Part print with two shaded views. Sizes in mm from the minimum x, y, z corner. Round coordinates to 2 decimals unless told otherwise and drop trailing zeros. Write each loop counter-clockwise with the first axis right and the second up, starting at its lowest first coordinate (ties: lowest second). Pieces come first, ordered by that corner, then holes. Notation, with made-up numbers: (-14, -29) - (-1, -29) arc R18 ccw to (-1, -19) - close; hole circle Ø4 at (56, 55.25). An arc over 180 degrees is marked (long way). Use one line per item in the form item = value. Start each with the question number.
Item 1: Drill centre lines: L1, parallel to Z at x = 125, y = 4.25; L2, parallel to X at y = 12, z = 80.5; L3, parallel to Z at x = 73, y = 8.5. Where is each one in solid material? Low to high.
Item 2: Band-saw the part on A-A, the plane z = 80.5. List the corners of the cut face in (x, y), and give its area (3 significant figures).
Item 3: Pin check, flat tips, straight feed: pin 1 (5 mm diameter, centred on y = 3, z = 27.5, fed in from -X); pin 2 (9.5 mm diameter, centred on x = 125, z = 80.5, fed in from -Y); pin 3 (3.5 mm diameter, centred on x = 125, z = 19.5, fed in from +Y). Stop position of each tip, or through.
Item 4: Band-saw the part on B-B, the plane x = 75. List the corners of the cut face in (y, z), and give its area (3 significant figures).
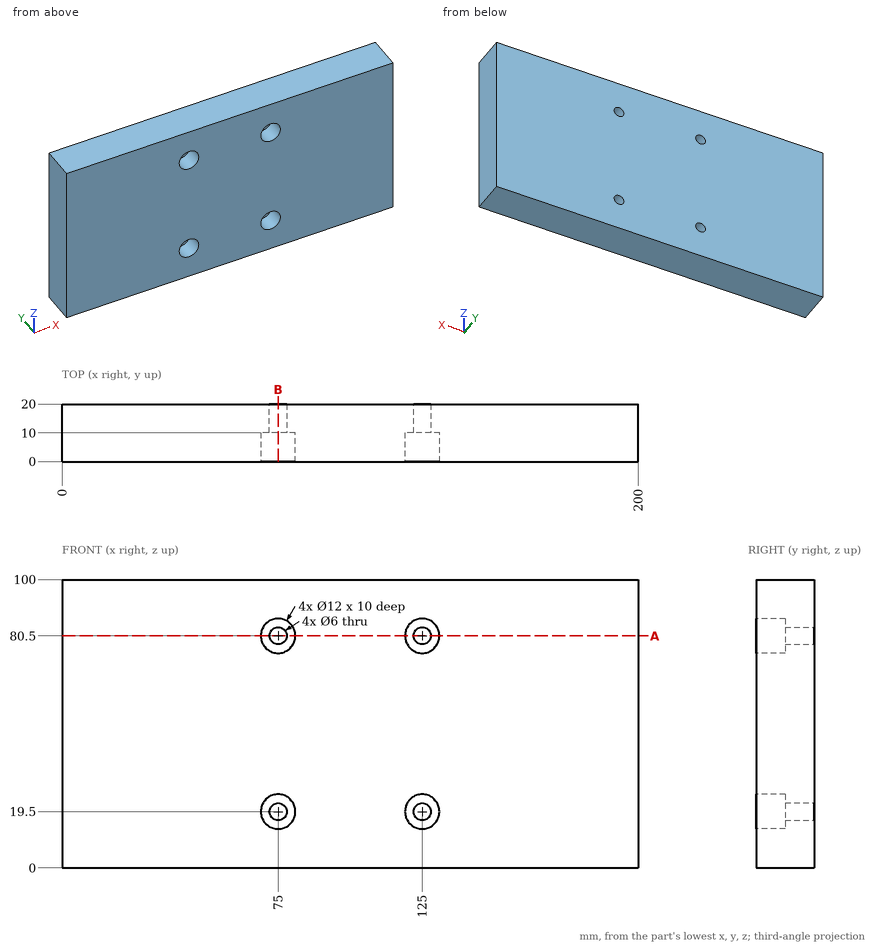
Determined:
q1.L1 = 0 to 13.5, 25.5 to 74.5, 86.5 to 100
q1.L2 = 0 to 72, 78 to 122, 128 to 200
q1.L3 = 0 to 13.84, 25.16 to 74.84, 86.16 to 100
q2.outline = (0, 0) - (69, 0) - (69, 10) - (72, 10) - (72, 20) - (0, 20) - close; (78, 10) - (81, 10) - (81, 0) - (119, 0) - (119, 10) - (122, 10) - (122, 20) - (78, 20) - close; (128, 10) - (131, 10) - (131, 0) - (200, 0) - (200, 20) - (128, 20) - close
q2.area = 3,640 mm²
q3.pin_1 = 0
q3.pin_2 = 10
q3.pin_3 = through
q4.outline = (0, 0) - (20, 0) - (20, 16.5) - (10, 16.5) - (10, 13.5) - (0, 13.5) - close; (0, 25.5) - (10, 25.5) - (10, 22.5) - (20, 22.5) - (20, 77.5) - (10, 77.5) - (10, 74.5) - (0, 74.5) - close; (0, 86.5) - (10, 86.5) - (10, 83.5) - (20, 83.5) - (20, 100) - (0, 100) - close
q4.area = 1,640 mm²
